Read the model definition and answer for the solid it produces. Units are mm, in the model's axes. A direction names the side the tool comes from. Coordinates: 2 decimals unless noted, no trailing zeros. Loops run counter-clockwise (first coordinate to the right, second up) from the corner with the lowest first, then second, coordinate; pieces in that order, holes last.
Autodesk Inventor part; units mm, degrees
ref_plane "DiagonalPlane1" through (23.57, -23.57, 0) normal (0.7071, 0.7071, 0) x (-0.7071, 0.7071, 0)
ref_plane "DiagonalPlane2" through (-23.57, -23.57, 0) normal (0.7071, -0.7071, 0) x (0.7071, 0.7071, 0)
ref_plane "YZ Plane" through (0, 0, 0) normal (1, 0, 0) x (0, 1, 0)
sketch "Sketch1" plane through (0, 0, 0) normal (0, 0, 1) x (1, 0, 0)
  line L0 (-28.5, 28.5) -> (28.5, 28.5)
  line L1 (28.5, 28.5) -> (28.5, -28.5)
  line L2 (28.5, -28.5) -> (-28.5, -28.5)
  line L3 (-28.5, -28.5) -> (-28.5, 28.5)
  line L4 (-28.5, 28.5) -> (28.5, -28.5) construction
  line L5 (28.5, 28.5) -> (-28.5, -28.5) construction
  line L6 (-23.57, 23.57) -> (23.57, 23.57) construction
  circle A0 centre (-23.57, 23.57) radius 2
  line L7 (0, 0) -> (0, 28.5) construction
  line L8 (-28.5, 0) -> (28.5, 0) construction
  circle A1 centre (23.57, 23.57) radius 2
  circle A2 centre (-23.57, -23.57) radius 2
  circle A3 centre (23.57, -23.57) radius 2
  dimension "d0" = 57
  dimension "d1" = 47.14
  dimension "d2" = 4
extrude "Extrusion1" add sketch "Sketch1" against normal blind 5
fillet "Fillet1" radius 4 4 edges at (28.5, -28.5, -2.5) (28.5, 28.5, -2.5) (-28.5, 28.5, -2.5) (-28.5, -28.5, -2.5)
sketch "Sketch2" plane through (0, 0, 0) normal (0, 0, 1) x (1, 0, 0)
  circle A0 centre (0, 0) radius 19.125
  dimension "d6" = 38.25
extrude "Extrusion2" add sketch "Sketch2" along normal blind 1.6
sketch "Sketch3" plane through (0, 0, 1.6) normal (0, 0, 1) x (1, 0, 0)
  circle A0 centre (0, 0) radius 9
  circle A1 centre (0, 0) radius 5
  circle A2 centre (0, 0) radius 8.75
  circle A3 centre (0, 0) radius 5.25
  dimension "d9" = 18
  dimension "d10" = 4
  dimension "d11" = 0.25
  dimension "d12" = 0.25
extrude "Extrusion3" cut sketch "Sketch3" against normal blind 0.25
sketch "Sketch4" plane through (0, 0, 1.6) normal (0, 0, 1) x (1, 0, 0)
  circle A0 centre (0, 0) radius 4
  dimension "d15" = 8
extrude "Extrusion4" add sketch "Sketch4" along normal blind 22
sketch "Sketch5" plane through (0, 0, 23.6) normal (0, 0, 1) x (1, 0, 0)
  circle A0 centre (0, 0) radius 4
  line L0 (-1.9365, 3.5) -> (1.9365, 3.5)
  line L1 (0, -4) -> (0, 3.5) construction
  dimension "d18" = 7.5
extrude "Extrusion5" cut sketch "Sketch5" against normal up to surface (22 mm away) contours L0 A0 picked at (-0.3981, 3.6058)
sketch "Sketch6" plane through (0, 0, -5) normal (0, 0, -1) x (-1, 0, 0)
  arc A0 (24.5, -28.5) -> (28.5, -24.5) centre (24.5, -24.5) ccw
  line L0 (28.5, -24.5) -> (28.5, 24.5)
  arc A1 (28.5, 24.5) -> (24.5, 28.5) centre (24.5, 24.5) ccw
  line L1 (24.5, 28.5) -> (-24.5, 28.5)
  arc A2 (-24.5, 28.5) -> (-28.5, 24.5) centre (-24.5, 24.5) ccw
  line L2 (-28.5, 24.5) -> (-28.5, -24.5)
  arc A3 (-28.5, -24.5) -> (-24.5, -28.5) centre (-24.5, -24.5) ccw
  line L3 (-24.5, -28.5) -> (24.5, -28.5)
  circle A4 centre (-23.57, -23.57) radius 2
  circle A5 centre (23.57, -23.57) radius 2
  circle A6 centre (-23.57, 23.57) radius 2
  circle A7 centre (23.57, 23.57) radius 2
  circle A8 centre (23.57, 23.57) radius 5.3152
  line L4 (0, 28.5) -> (0, -28.5)
  line L5 (28.5, 0) -> (-28.5, 0)
  circle A9 centre (23.57, -23.57) radius 5.3152
  circle A10 centre (-23.57, 23.57) radius 5.3152
  circle A11 centre (-23.57, -23.57) radius 5.3152
  point P0 (0, 0)
  point P1 (28.5, 21.5834)
  point P2 (21.5834, 28.5)
  point P3 (-21.5834, 28.5)
  point P4 (-28.5, 21.5834)
  point P5 (-28.5, -21.5834)
  point P6 (-21.5834, -28.5)
  point P7 (21.5834, -28.5)
  point P8 (28.5, -21.5834)
extrude "Extrusion6" add sketch "Sketch6" along normal blind 41 contours L3 L4 L5 L0 A9 | L3 A11 L2 L5 L4 | L5 L2 A10 L1 L4 | L4 L1 A8 L0 L5
fillet "Fillet2" radius 2 8 edges at (-28.5, 21.5834, -25.5) (-21.5834, 28.5, -25.5) (-28.5, -21.5834, -25.5) (-21.5834, -28.5, -25.5) (21.5834, 28.5, -25.5) (28.5, 21.5834, -25.5) (28.5, -21.5834, -25.5) (21.5834, -28.5, -25.5)
sketch "Sketch8" plane through (-24.5, 28.5, 0) normal (0, 1, 0) x (1, 0, 0)
  line L0 (41.3672, 46) -> (7.6328, 46)
  line L1 (35.5, 46) -> (13.5, 46)
  line L2 (13.5, 46) -> (13.5, 29)
  line L3 (13.5, 29) -> (35.5, 29)
  line L4 (35.5, 29) -> (35.5, 46)
  line L5 (24.5, 0) -> (24.5, 46) construction
  point P0 (24.5, 29)
  point P1 (13.5, 46)
  dimension "d24" = 22
  dimension "d25" = 17
extrude "Extrusion7" add sketch "Sketch8" along normal blind 9
chamfer "Chamfer1" distance 4 angle 45 2 edges at (11, 37.5, -37.5) (-11, 37.5, -37.5)
sketch "DiagonalProfile" plane through (0, 0, 0) normal (0, 0, 1) x (1, 0, 0)
  circle A0 centre (-23.57, -23.57) radius 2
  circle A1 centre (23.57, 23.57) radius 2
  line L0 (-23.57, -23.57) -> (23.57, 23.57)
  circle A2 centre (23.57, -23.57) radius 2
  circle A3 centre (-23.57, 23.57) radius 2
  line L1 (23.57, -23.57) -> (-23.57, 23.57)
  point P0 (0, 0)
ref_plane "DiagonalPlane1" through (23.57, -23.57, 0) normal (0.7071, 0.7071, 0) x (-0.7071, 0.7071, 0)
ref_plane "DiagonalPlane2" through (-23.57, -23.57, 0) normal (0.7071, -0.7071, 0) x (0.7071, 0.7071, 0)
properties part number "SouluckNema23-0.7N-24V"
Item 1: Determine the mould class of faces 6 (the face through (0, -4, 12)), 7 (the face through (-27.618, 18.526, -25.787)), 8 (the face through (19.749, 19.875, -25.213)) for opening direction Y: released by +Y, released by -Y, zero draft, split by the parting line, or undercut.
Numbers:
face 6: split by the parting line
face 7: released by +Y
face 8: undercut
Item 2: Given pin 1 (8 mm diameter, centred on x = -20.5, y = 13, fed in from +Z); pin 2 (23 mm diameter, centred on x = 1.5, z = -21.5, fed in from +Y); pin 3 (5 mm diameter, centred on x = -23.57, y = 23.57, fed in from -Z); pin 4 (2 mm diameter, centred on y = 21, z = -31, fed in from +X), each flat-ended and moving along its own axis, determine where each tip first touches the part or whether it passes through.
Numbers:
pin 1: stops at z = 0
pin 2: stops at y = 37.5
pin 3: stops at z = -5
pin 4: stops at x = 19.63
Item 3: Which of the six approach directions +Z, -Z, +X, -X, +Y, -Y give full straight-line access (tool end or side, diameter ignored) to faces 1 (the face through (-18.526, -27.618, -25.787)), 2 (the face through (4, -4, 1.6)), 3 (the face through (27.618, -18.526, -25.787)), 4 (the face through (18.526, 27.618, -25.787)), 5 (the face through (-19.875, 19.749, -25.213))?
Numbers:
face 1: -Z, -X
face 2: +Z
face 3: -Z, -Y
face 4: -Z, +X
face 5: -Z
Item 4: Find the intervals of material crossed by line 1 along Y through (x, z) = (0, 1.55) (3 decimals); line 2 along Y through (x, z) = (23.57, -3.7); line 3 along Y through (x, z) = (-23, -2), in increasing order.
Numbers:
line 1: y = -19.125 to -9, -8.75 to -5.25, -5 to 5, 5.25 to 8.75, 9 to 19.125
line 2: y = -28.5 to -25.57, -21.57 to 21.57, 25.57 to 28.5
line 3: y = -28.5 to -25.49, -21.65 to 21.65, 25.49 to 28.5
Item 5: A cutting plane is placed at A-A on y = 23.57. Determine the outline of the cut face in (x, z), then the cut area to 3 significant figures.
Numbers:
outline: (-28.5, -5) - (-25.57, -5) - (-25.57, 0) - (-28.5, 0) - close; (-21.57, -5) - (-18.25, -5) - (-18.25, -46) - (18.25, -46) - (18.25, -5) - (21.57, -5) - (21.57, 0) - (-21.57, 0) - close; (25.57, -5) - (28.5, -5) - (28.5, 0) - (25.57, 0) - close
area: 1,740 mm2
Item 6: A cutting plane is placed at C-C on y = 0. Determine the outline of the cut face in (x, z) (3 decimals), then the cut area to 3 significant figures.
Numbers:
outline: (-28.5, -46) - (28.5, -46) - (28.5, 0) - (19.125, 0) - (19.125, 1.6) - (9, 1.6) - (9, 1.35) - (8.75, 1.35) - (8.75, 1.6) - (5.25, 1.6) - (5.25, 1.35) - (5, 1.35) - (5, 1.6) - (4, 1.6) - (4, 23.6) - (-4, 23.6) - (-4, 1.6) - (-5, 1.6) - (-5, 1.35) - (-5.25, 1.35) - (-5.25, 1.6) - (-8.75, 1.6) - (-8.75, 1.35) - (-9, 1.35) - (-9, 1.6) - (-19.125, 1.6) - (-19.125, 0) - (-28.5, 0) - close
area: 2,860 mm2
